Model file for the job. Use its own axes, mm. Face numbers are marked on the shaded views. A direction names the side the tool comes from. Give positions to 0.01 mm unless a question says otherwise; leave off trailing zeros. Order: outer loops, then holes, each group sorted by start corner. A loop starts at its lowest first (then second) coordinate and runs counter-clockwise, first axis right, second up. Notation, with made-up numbers: M 27.5,0.5 L 64.5,0.5 A11 ccw 64.5,17.5 Z; hole C 54.5,-30 d3. An arc over 180 degrees is marked long. Return JSON: item names as keys, results as strings. Group by question number.
1. 3-axis set-ups, long thin cutter, end or side, ignore diameter. For the marked faces 4, 5, 6 and 7: which of +Z, -Z, +X, -X, +Y, -Y reach the whole face in a straight line?
2. Slice it at D-D on y = 1.75. List the corners of the cut face in (x, z).
3. Slice it at B-B on y = 0.2. Give the number of separate pieces and of enclosed holes in the cut face, then the cut area to 3 significant figures.
4. Slice it at A-A on x = -0.25. List the corners of the cut face in (y, z).
5. Wall check: probe 1 along X at (y, z) = (-0.5, 2.5); probe 2 along Y at (x, z) = (0.25, 1.75); probe 3 along X at (y, z) = (-1.05, 6.5). Give the ranges that are in metal, low to high. Write a range as [from, to].
6. Slice it at C-C on z = 1.5. List the corners of the cut face in (x, y), then the cut area to 3 significant figures.
7. Two-plate mould, pull along Y, no slides. Class the marked faces 1, 2 and 3: released by +Y, released by -Y, zero draft, split by the parting line, or undercut.
8. Pin check, flat tips, straight feed: pin 1 (1.6 mm diameter, centred on x = 0, z = 4, fed in from -Y); pin 2 (0.5 mm diameter, centred on x = 2.5, z = 0.5, fed in from +Y); pin 3 (0.5 mm diameter, centred on y = 0.5, z = 0.5, fed in from +X). Stop position of each tip, or through.
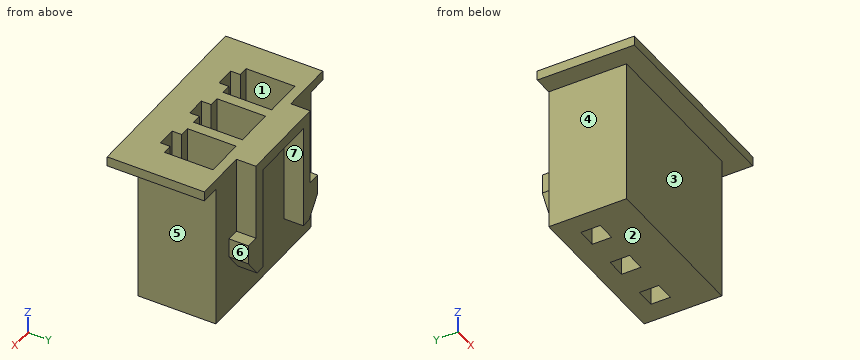
Autodesk Inventor part; units mm, degrees
ref_plane "YZ Plane" through (0, 0, 0) normal (1, 0, 0) x (0, 1, 0)
ref_plane "XZ Plane" through (0, 0, 0) normal (0, 1, 0) x (-1, 0, 0)
ref_plane "XY Plane" through (0, 0, 0) normal (0, 0, 1) x (1, 0, 0)
sketch "Esquisse1" plane through (0, 0, 0) normal (0, 0, 1) x (1, 0, 0)
  line L0 (-4.12, -2) -> (4.12, -2)
  line L1 (4.12, -2) -> (4.12, 2)
  line L2 (4.12, 2) -> (-4.12, 2)
  line L3 (-4.12, 2) -> (-4.12, -2)
  line L4 (-4.12, -2) -> (4.12, 2) construction
  line L5 (4.12, -2) -> (-4.12, 2) construction
  point P0 (0, 0)
  dimension "d0" = 8.24
  dimension "d1" = 4
extrude "Embase" add sketch "Esquisse1" along normal blind 7.5
sketch "Esquisse2" plane through (0, 0, 7.5) normal (0, 0, 1) x (1, 0, 0)
  line L0 (-5.12, -3) -> (5.12, -3)
  line L1 (5.12, -3) -> (5.12, 2)
  line L2 (5.12, 2) -> (-5.12, 2)
  line L3 (-5.12, 2) -> (-5.12, -3)
  line L4 (-5.12, -3) -> (5.12, 2) construction
  line L5 (5.12, -3) -> (-5.12, 2) construction
  line L6 (4.12, 2) -> (-4.12, 2)
  line L7 (4.12, -2) -> (4.12, 2)
  point P0 (0, -0.5)
  point P1 (0, 0)
  point P2 (0, -0.5)
  dimension "d5" = 5
  dimension "d9" = 1
extrude "Epaulement" add sketch "Esquisse2" along normal blind 0.5
sketch "Esquisse4" plane through (-4.12, 2, 0) normal (0, 1, 0) x (1, 0, 0)
  line L0 (5.87, -2) -> (5.87, -7.4)
  line L1 (5.87, -7.4) -> (2.37, -7.4)
  line L2 (2.37, -7.4) -> (2.37, -2)
  line L3 (2.37, -2) -> (1.87, -2)
  line L4 (1.87, -2) -> (1.12, -3)
  line L5 (1.12, -4) -> (1.77, -4)
  line L6 (1.77, -4) -> (1.77, -8)
  line L7 (1.77, -8) -> (6.47, -8)
  line L8 (6.47, -8) -> (6.47, -4)
  line L9 (6.47, -4) -> (7.12, -4)
  line L10 (7.12, -3) -> (6.37, -2)
  line L11 (6.37, -2) -> (5.87, -2)
  line L12 (8.24, 0) -> (0, 0)
  line L13 (9.24, -8) -> (-1, -8) construction
  line L14 (7.12, -3) -> (7.12, -4)
  line L15 (1.12, -4) -> (1.12, -3)
  point P0 (4.12, 0)
  point P1 (4.12, -7.4)
  point P2 (4.12, 0)
  dimension "d10" = 0.6
  dimension "d11" = 0.6
  dimension "Entre_clip" = 3.5
  dimension "d13" = 6
  dimension "d14" = 4
  dimension "d15" = 1
  dimension "d16" = 0.6
  dimension "d18" = 0.5
  dimension "d21" = 0.65
extrude "Clip" add sketch "Esquisse4" along normal blind 1
sketch "Esquisse5" plane through (0, 0, 8) normal (0, 0, 1) x (1, 0, 0)
  line L0 (3.54, -1) -> (3.54, 1.5)
  line L1 (3.54, 1.5) -> (1.54, 1.5)
  line L2 (1.54, 1.5) -> (1.54, -1)
  line L3 (5.12, -3) -> (5.12, 2)
  line L4 (2.54, 1.25) -> (2.54, -1.75) construction
  line L5 (3.04, -1) -> (3.04, -1.4998)
  line L6 (3.04, -1.4998) -> (2.04, -1.4998)
  line L7 (2.04, -1.4998) -> (2.04, -1)
  line L8 (1.54, -1) -> (2.04, -1)
  line L9 (3.04, -1) -> (3.54, -1)
  line L10 (5.12, 2) -> (2.35, 2)
  point P0 (0, 0)
  point P1 (2.04, 1.5)
  point P2 (3.54, 0.25)
  point P3 (5.12, -0.5)
  point P4 (2.54, -1.713)
  point P5 (2.54, -1.4998)
  point P6 (2.54, 1.5)
  dimension "d22" = 2.58
  dimension "d24" = 2.5
  dimension "d34" = 0.4998
  dimension "d35" = 1
  dimension "d36" = 2
  dimension "d37" = 0.5
extrude "Extrusion4" cut sketch "Esquisse5" against normal blind 7
sketch "Esquisse6" plane through (0, 0, 1) normal (0, 0, 1) x (1, 0, 0)
  line L0 (2.04, 0) -> (3.04, 0)
  line L1 (3.04, 0) -> (3.04, 1)
  line L2 (3.04, 1) -> (2.04, 1)
  line L3 (2.04, 1) -> (2.04, 0)
  line L4 (2.04, -1) -> (1.54, -1)
  line L5 (1.54, 1.5) -> (3.54, 1.5)
  line L6 (3.04, -1.4998) -> (2.04, -1.4998)
  point P0 (0, 0)
  point P1 (2.54, 1)
  point P2 (2.96, -1.75)
  point P3 (2.54, 0)
  point P4 (2.54, -1.4998)
  dimension "d29" = 1
  dimension "d30" = 1
  dimension "d38" = 0.5
extrude "Extrusion5" cut sketch "Esquisse6" against normal through all
pattern_linear "Réseau rectangulaire1" count 3 spacing 2.54 along (-1, 0, 0) of "Extrusion4", "Extrusion5"
equation "\"d11\" = d10"
equation "\"Entre_clip\" = 0.116667 * Nb_broche"
equation "\"d16\" = d11"
equation "\"Pas\" = 2.54"
properties part number "Connecteur JST 3 Broches Male" material "Plastique ABS"
Result:
{
 "1": {"face 4": "-Z, -X, +Y, -Y", "face 5": "-Z, +X, +Y, -Y", "face 6": "+Z, -Z, +X, +Y", "face 7": "-Z, +Y"},
 "2": {"outline": "M -5.12,7.5 L -4.12,7.5 L -4.12,0 L 4.12,0 L 4.12,7.5 L 5.12,7.5 L 5.12,8 L -5.12,8 Z"},
 "3": {"separate pieces": "4", "enclosed holes": "0", "area": "21.9 mm2"},
 "4": {"outline": "M -3,7.5 L -2,7.5 L -2,0 L 0,0 L 0,1 L -1.5,1 L -1.5,8 L -3,8 Z; M 1,0 L 2,0 L 2,7.4 L 3,7.4 L 3,8 L 1.5,8 L 1.5,1 L 1,1 Z"},
 "5": {"probe 1": "x = [-4.12, -3.54], [-1.54, -1], [1, 1.54], [3.54, 4.12]", "probe 2": "y = [-2, -1.5], [1.5, 2]", "probe 3": "x = [-4.12, -3.04], [-2.04, -0.5], [0.5, 2.04], [3.04, 4.12]"},
 "6": {"outline": "M -4.12,-2 L 4.12,-2 L 4.12,2 L -4.12,2 Z; hole M -3.54,-1 L -3.04,-1 L -3.04,-1.5 L -2.04,-1.5 L -2.04,-1 L -1.54,-1 L -1.54,1.5 L -3.54,1.5 Z; hole M -1,-1 L -0.5,-1 L -0.5,-1.5 L 0.5,-1.5 L 0.5,-1 L 1,-1 L 1,1.5 L -1,1.5 Z; hole M 1.54,-1 L 2.04,-1 L 2.04,-1.5 L 3.04,-1.5 L 3.04,-1 L 3.54,-1 L 3.54,1.5 L 1.54,1.5 Z", "area": "16.5 mm2"},
 "7": {"face 1": "undercut", "face 2": "zero draft", "face 3": "released by -Y"},
 "8": {"pin 1": "stops at y = -2", "pin 2": "stops at y = 2", "pin 3": "stops at x = 4.12"}
}
